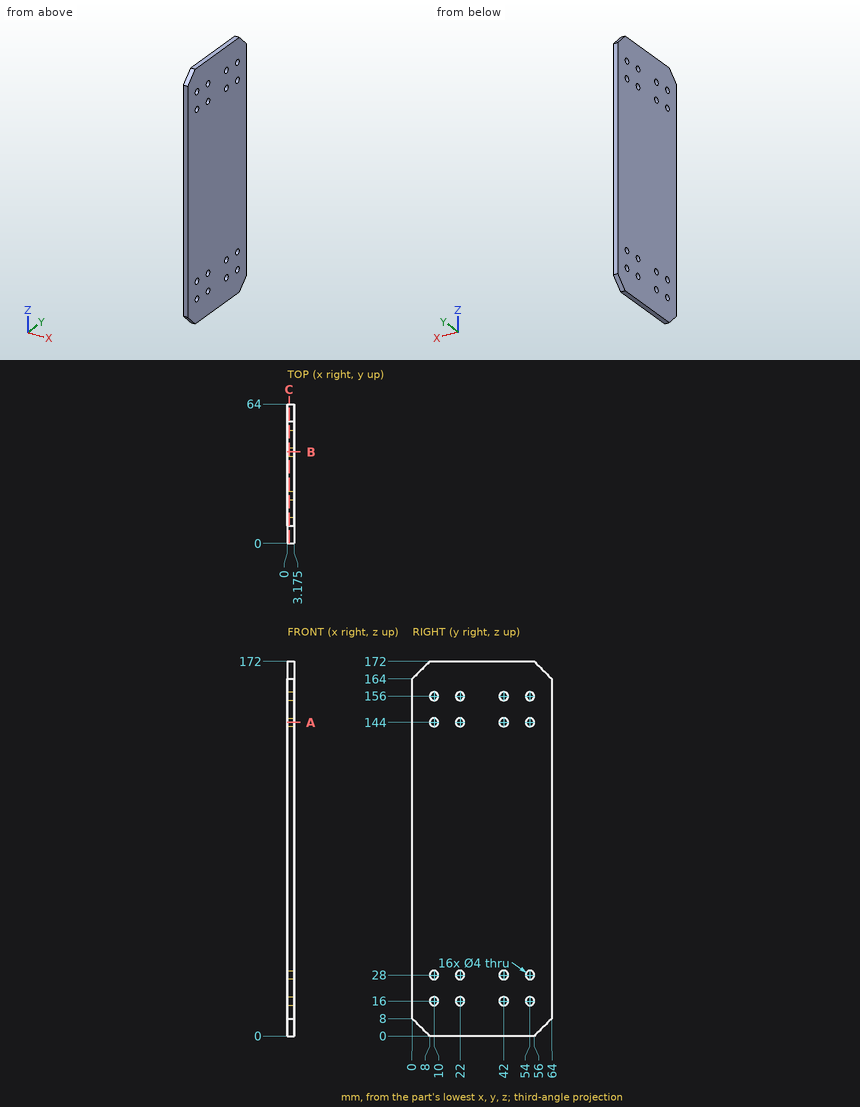
Geometry check sheet. Reference: drawing and pictorial views, mm from the part's lowest x, y, z. Coordinates: 2 decimals unless noted, no trailing zeros. Order: outer loops, then holes, each group sorted by start corner. A loop starts at its lowest first (then second) coordinate and runs counter-clockwise, first axis right, second up. Notation, with made-up numbers: M 21,70.5 L 75,70.5 A22 ccw 75,99.5 Z; hole C 22,-38.5 d2. An arc over 180 degrees is marked long. Write each question's results on one line, items separated by ' | '. Start each with the question number.
1. Cross-section at B-B on y = 42. Record the cut outline in (x, z) (3 decimals).
2. Cross-section at A-A on z = 144. Record the cut outline in (x, y) (3 decimals), and give its area (3 significant figures).
3. Cross-section at C-C on x = 0.8. State how many separate pieces and enclosed holes the cut face has, and give its area (3 significant figures).
4. Material ranges on probe 1 along Y at (x, z) = (1.6, 144); probe 2 along Z at (x, y) = (2.75, 43.5), recorded low to high.
Checks:
1) outline: M 0,0 L 3.175,0 L 3.175,14 L 0,14 Z; M 0,18 L 3.175,18 L 3.175,26 L 0,26 Z; M 0,30 L 3.175,30 L 3.175,142 L 0,142 Z; M 0,146 L 3.175,146 L 3.175,154 L 0,154 Z; M 0,158 L 3.175,158 L 3.175,172 L 0,172 Z
2) outline: M 0,0 L 3.175,0 L 3.175,8 L 0,8 Z; M 0,12 L 3.175,12 L 3.175,20 L 0,20 Z; M 0,24 L 3.175,24 L 3.175,40 L 0,40 Z; M 0,44 L 3.175,44 L 3.175,52 L 0,52 Z; M 0,56 L 3.175,56 L 3.175,64 L 0,64 Z | area: 152 mm²
3) separate pieces: 1 | enclosed holes: 16 | area: 10,700 mm²
4) probe 1: y = 0 to 8, 12 to 20, 24 to 40, 44 to 52, 56 to 64 | probe 2: z = 0 to 14.68, 17.32 to 26.68, 29.32 to 142.68, 145.32 to 154.68, 157.32 to 172
